```python
from build123d import *

# Parameters (mm, degrees)
SKETCH_1_R          = 30
EXTRUDE_1_DEPTH     = 8
SKETCH_2_R          = 1.6
CUT_EXTRUDE_1_DEPTH = 15
SKETCH_3_R          = 1.5
CUT_EXTRUDE_2_DEPTH = 8
SKETCH_4_R          = 3
CUT_EXTRUDE_3_DEPTH = 1
SKETCH_5_R          = 1.5
CUT_EXTRUDE_4_DEPTH = 4


with BuildPart() as part:
    # 草图1 → 凸台-拉伸1 (new body)
    with BuildSketch(Plane(origin=(0, 0, 0), x_dir=(1, 0, 0), z_dir=(0, 1, 0))):
        Circle(SKETCH_1_R)
    extrude(amount=EXTRUDE_1_DEPTH)

    # 草图2 → 切除-拉伸1 (cut)
    with BuildSketch(Plane(origin=(0, 8, 0), x_dir=(1, 0, 0), z_dir=(0, 1, 0))):
        with Locations((0, 13.5)):
            Circle(SKETCH_2_R)
        with Locations((11.691342951, -6.75)):
            Circle(SKETCH_2_R)
        with Locations((-11.691342951, -6.75)):
            Circle(SKETCH_2_R)
    extrude(amount=-CUT_EXTRUDE_1_DEPTH, mode=Mode.SUBTRACT)

    # 草图3 → 切除-拉伸2 (cut)
    with BuildSketch(Plane(origin=(0, 8, 0), x_dir=(1, 0, 0), z_dir=(0, 1, 0))):
        with Locations((17.320508076, 10)):
            Circle(SKETCH_3_R)
        with Locations((0, -20)):
            Circle(SKETCH_3_R)
        with Locations((-17.320508076, 10)):
            Circle(SKETCH_3_R)
    extrude(amount=-CUT_EXTRUDE_2_DEPTH, mode=Mode.SUBTRACT)

    # 草图4 → 切除-拉伸3 (cut)
    with BuildSketch(Plane(origin=(0, 8, 0), x_dir=(1, 0, 0), z_dir=(0, 1, 0))):
        with Locations((0, 13.5)):
            Circle(SKETCH_4_R)
        with Locations((11.691342951, -6.75)):
            Circle(SKETCH_4_R)
        with Locations((-11.691342951, -6.75)):
            Circle(SKETCH_4_R)
    extrude(amount=-CUT_EXTRUDE_3_DEPTH, mode=Mode.SUBTRACT)

    # 草图5 → 切除-拉伸4 (cut)
    with BuildSketch(Plane.XZ):
        Polygon((-14.722431864, -10), (-16.02146997, -7.75), (-18.619546181, -7.75), (-19.918584287, -10), (-18.619546181, -12.25), (-16.02146997, -12.25), align=None)
        with Locations((-17.320508076, -10)):
            Circle(SKETCH_5_R, mode=Mode.SUBTRACT)
        Polygon((16.02146997, -7.75), (14.722431864, -10), (16.02146997, -12.25), (18.619546181, -12.25), (19.918584287, -10), (18.619546181, -7.75), align=None)
        with Locations((17.320508076, -10)):
            Circle(SKETCH_5_R, mode=Mode.SUBTRACT)
        Polygon((1.299038106, 22.25), (-1.299038106, 22.25), (-2.598076211, 20), (-1.299038106, 17.75), (1.299038106, 17.75), (2.598076211, 20), align=None)
    extrude(amount=-CUT_EXTRUDE_4_DEPTH, mode=Mode.SUBTRACT)


solid = part.part
```
Geometry: final body of the model. Coordinates: model frame, mm. A direction names the side the tool comes from. Coordinates: 2 decimals unless noted, no trailing zeros. Loops run counter-clockwise (first coordinate to the right, second up) from the corner with the lowest first, then second, coordinate; pieces in that order, holes last. Notation, with made-up numbers: M 16,4.5 L 55,4.5 A22 cw 55,31.5 Z; hole C 64,5 d11. An arc over 180 degrees is marked long. Put each result on its own line as item: value.
(1) Cut plane B-B on x = 0. Return the cut outline in (y, z), then the cut area to 3 significant figures.
Answer sheet:
outline: M 0,-30 L 8,-30 L 8,-16.5 L 7,-16.5 L 7,-15.1 L 0,-15.1 Z; M 0,-11.9 L 7,-11.9 L 7,-10.5 L 8,-10.5 L 8,18.5 L 4,18.5 L 4,17.75 L 0,17.75 Z; M 0,22.25 L 4,22.25 L 4,21.5 L 8,21.5 L 8,30 L 0,30 Z
area: 422 mm^2
(2) Cut plane A-A on y = 2. Return the cut outline in (x, z), then the cut area to 3 significant figures.
Answer sheet:
outline: C 0,0 d60; hole M -19.92,-10 L -18.62,-12.25 L -16.02,-12.25 L -14.72,-10 L -16.02,-7.75 L -18.62,-7.75 Z; hole C -11.69,6.75 d3.2; hole M -2.6,20 L -1.3,17.75 L 1.3,17.75 L 2.6,20 L 1.3,22.25 L -1.3,22.25 Z; hole C 0,-13.5 d3.2; hole C 11.69,6.75 d3.2; hole M 14.72,-10 L 16.02,-12.25 L 18.62,-12.25 L 19.92,-10 L 18.62,-7.75 L 16.02,-7.75 Z
area: 2,750 mm^2
(3) Access query for faces 1 (the face through (-0.65, 7.51, -10.57)), 2 (the face through (-15.38, 1.97, -11.14)), 3 (the face through (11.3, 3.5, 8.3)). Directions: +Z, -Z, +X, -X, +Y, -Y. A direction counts if a zero-diameter tool reaches every point of the face in a straight line with its end or side. Return the directions, or none.
Answer sheet:
face 1: +Y
face 2: -Y
face 3: +Y, -Y
(4) Material intervals for probe 1 along Z at (x, y) = (0, 2); probe 2 along X at (y, z) = (1.5, 6.75); probe 3 along X at (y, z) = (6.35, -10), sorted ascending.
Answer sheet:
probe 1: z = -30 to -15.1, -11.9 to 17.75, 22.25 to 30
probe 2: x = -29.23 to -13.29, -10.09 to 10.09, 13.29 to 29.23
probe 3: x = -28.28 to -18.82, -15.82 to 15.82, 18.82 to 28.28
(5) First-contact query: pin 1 (1.9 mm diameter, centred on x = 11.69, z = 6.75, fed in from +Y); pin 2 (1 mm diameter, centred on y = 5, z = 17.5, fed in from +X); pin 3 (4 mm diameter, centred on x = -12.5, y = 4.5, fed in from -Z); pin 4 (1.3 mm diameter, centred on x = -16.5, y = 2.5, fed in from +Z). Flat tips, straight axial feed; report the tip coordinate or a pass-through.
Answer sheet:
pin 1: passes through
pin 2: stops at x = 24.72
pin 3: stops at z = -28.1
pin 4: stops at z = 25.47
(6) Cut plane C-C on z = 6.75. Return the cut outline in (x, y), then the cut area to 3 significant figures.
Answer sheet:
outline: M -29.23,0 L -13.29,0 L -13.29,7 L -14.69,7 L -14.69,8 L -29.23,8 Z; M -10.09,0 L 10.09,0 L 10.09,7 L 8.69,7 L 8.69,8 L -8.69,8 L -8.69,7 L -10.09,7 Z; M 13.29,0 L 29.23,0 L 29.23,8 L 14.69,8 L 14.69,7 L 13.29,7 Z
area: 411 mm^2
(7) Draft query along Z for faces 4 (the face through (18.75, 6.03, -10.45)), 5 (the face through (0, 0, 0)), 6 (the face through (19.26, 1.97, -11.14)). Return one class per face: pulls with the +Z half, pulls with the -Z half, needs draft (parallel to the pull), parting line crosses it, or undercut.
Answer sheet:
face 4: undercut
face 5: needs draft
face 6: undercut
(8) Cut plane D-D on z = -13.5. Return the cut outline in (x, y), then the cut area to 3 significant figures.
Answer sheet:
outline: M -26.79,0 L -1.6,0 L -1.6,7 L -3,7 L -3,8 L -26.79,8 Z; M 1.6,0 L 26.79,0 L 26.79,8 L 3,8 L 3,7 L 1.6,7 Z
area: 400 mm^2
